from build123d import *

# Parameters (mm, degrees)
F1_DEPTH = 7.874
F0_R     = 2.286
F2_DEPTH = 2.159
F3_W     = 17.78
F3_H     = 2.54
F4_DEPTH = 43.18


with BuildPart() as f1:
    # F0 (on Top) → F1 (new body)
    with BuildSketch(Plane.XY):
        with BuildLine():
            ThreePointArc((-24.7015, -6.985), (-23.7715640303, -9.2300640303), (-21.5265, -10.16))
            Line((-21.5265, -10.16), (24.7015, -10.16))
            Line((24.7015, -10.16), (24.7015, -7.62))
            Line((24.7015, -7.62), (-21.463, -7.62))
            ThreePointArc((-21.463, -7.62), (-22.5855320151, -7.1550320151), (-23.0505, -6.0325))
            Line((-23.0505, -6.0325), (-23.0505, 6.0325))
            ThreePointArc((-23.0505, 6.0325), (-22.5855320151, 7.1550320151), (-21.463, 7.62))
            Line((-21.463, 7.62), (24.7015, 7.62))
            Line((24.7015, 7.62), (24.7015, 10.16))
            Line((24.7015, 10.16), (-21.5265, 10.16))
            ThreePointArc((-21.5265, 10.16), (-23.7715640303, 9.2300640303), (-24.7015, 6.985))
            Line((-24.7015, 6.985), (-24.7015, -6.985))
        make_face()
    extrude(amount=F1_DEPTH)

    # F0 (on Top) → F2 (join)
    with BuildSketch(Plane.XY):
        with BuildLine():
            Line((-21.463, -7.62), (24.7015, -7.62))
            Line((24.7015, -7.62), (24.7015, 7.62))
            Line((24.7015, 7.62), (-21.463, 7.62))
            ThreePointArc((-21.463, 7.62), (-22.5855320151, 7.1550320151), (-23.0505, 6.0325))
            Line((-23.0505, 6.0325), (-23.0505, -6.0325))
            ThreePointArc((-23.0505, -6.0325), (-22.5855320151, -7.1550320151), (-21.463, -7.62))
        make_face()
        with Locations((2.9845, 0)):
            Circle(F0_R, mode=Mode.SUBTRACT)
        with Locations((2.9845, 0)):
            Circle(F0_R)
    extrude(amount=F2_DEPTH)

    # F3 (on face) → F4 (cut)
    with BuildSketch(Plane.YZ.offset(24.7015)):
        with Locations((0, 3.429)):
            Rectangle(F3_W, F3_H)
    extrude(amount=-F4_DEPTH, mode=Mode.SUBTRACT)


solid = f1.part
The model under review builds one solid part; all positions refer to its coordinate system, in mm. A direction names the side the tool comes from. Round coordinates to 2 decimals unless told otherwise and drop trailing zeros. Loops run counter-clockwise (first coordinate to the right, second up) from the corner with the lowest first, then second, coordinate; pieces in that order, holes last. Notation, with made-up numbers: M 88.25,28 L 134.25,28 A5 ccw 134.25,33 Z; hole C 89.5,19 d8. An arc over 180 degrees is marked long. Answer as a JSON object with one key per item and string values.
Item 1: We need section C-C, the plane x = 15. State the section outline as (y, z) points.
Check sheet entries:
{"outline": "M -10.16,0 L 10.16,0 L 10.16,7.87 L 7.62,7.87 L 7.62,4.7 L 8.89,4.7 L 8.89,2.16 L -8.89,2.16 L -8.89,4.7 L -7.62,4.7 L -7.62,7.87 L -10.16,7.87 Z"}
Item 2: The part is to be moulded in two halves that separate along Y. For faces 1 (the face through (-24.702, 0, 4)), 2 (the face through (-18.478, 8, 3)), 3 (the face through (-23.8, -9.2, 3.9)), say which applies: +Y half, -Y half, draft (parallel to the pull), parting line (faces both ways), or undercut.
Check sheet entries:
{"face 1": "draft", "face 2": "undercut", "face 3": "-Y half"}
Item 3: For line 1 along Z through (x, y) = (-4, 8.5); line 2 along Y through (x, z) = (-7, 5); line 3 along Y through (x, z) = (-4, 2.5), list the stretches that pass through material, from the lowest coordinate up.
Check sheet entries:
{"line 1": "0 to 2.16, 4.7 to 7.87", "line 2": "-10.16 to -7.62, 7.62 to 10.16", "line 3": "-10.16 to -8.89, 8.89 to 10.16"}
Item 4: Tool access review of faces 4 (the face through (-22.6, 7.14, 4.98)), 5 (the face through (1, 0, 2.159)), 6 (the face through (24.702, 0, 2)): name each direction out of +Z, -Z, +X, -X, +Y, -Y from which nothing blocks a thin tool from reaching the whole face with its end or side.
Check sheet entries:
{"face 4": "+Z, +X", "face 5": "+X", "face 6": "+Z, -Z, +X, +Y, -Y"}
Item 5: Clearance check with flat-ended pins moving along their axes: P1, Ø5.5, axis at x = 3, y = -1, coming from the +Z side; P2, Ø1.5, axis at y = -1.5, z = 5, coming from the +X side; P3, Ø1.4, axis at y = -8, z = 3, coming from the +X side. State where each tip first meets the part, or that it passes through.
Check sheet entries:
{"P1": "z = 2.16", "P2": "x = -23.05", "P3": "x = -18.48"}
Item 6: We need section B-B, the plane y = -5.5. State the section outline as (x, z) points.
Check sheet entries:
{"outline": "M -24.7,0 L 24.7,0 L 24.7,2.16 L -23.05,2.16 L -23.05,7.87 L -24.7,7.87 Z"}
